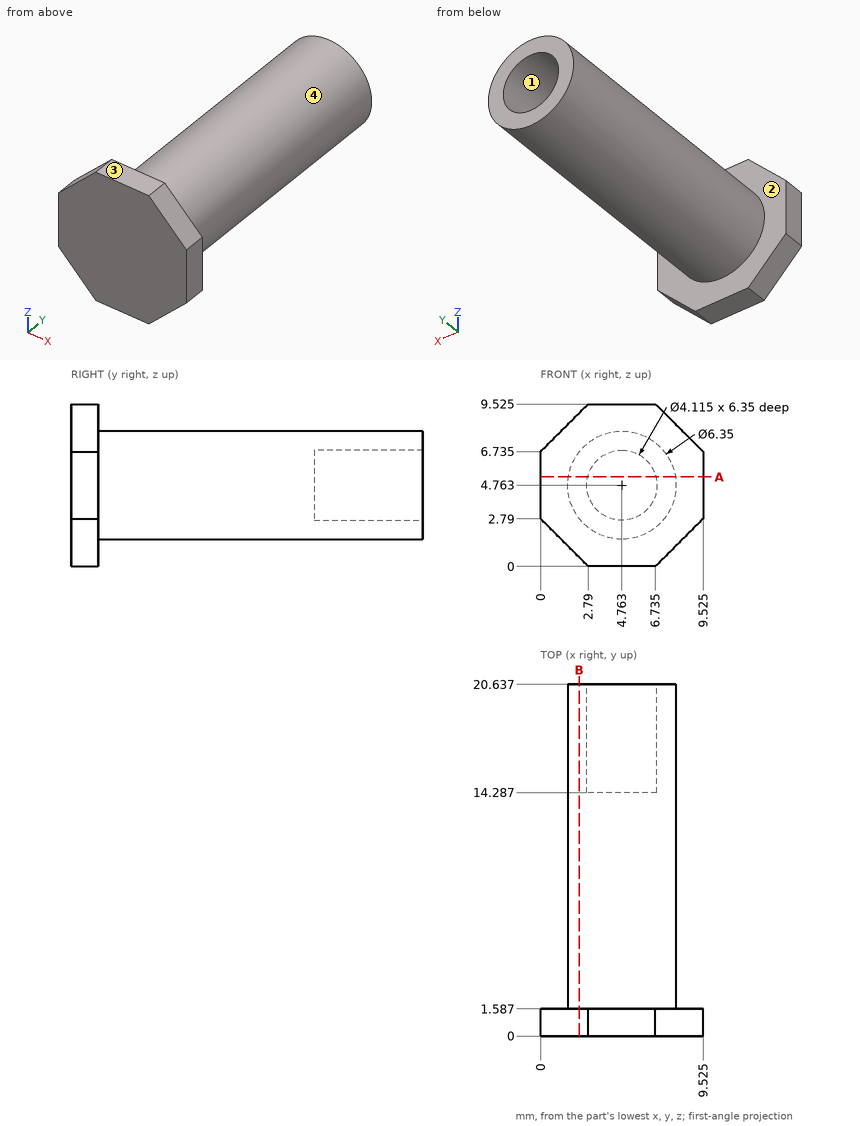
Geometry check sheet. Reference: drawing and pictorial views, mm from the part's lowest x, y, z. Give positions to 0.01 mm unless a question says otherwise; leave off trailing zeros. Order: outer loops, then holes, each group sorted by start corner. A loop starts at its lowest first (then second) coordinate and runs counter-clockwise, first axis right, second up. Notation, with made-up numbers: M -22.5,-20 L 22.5,-20 A29 ccw 22.5,8 Z; hole C 0.25,-35.75 d1. An arc over 180 degrees is marked long. Answer in a Markdown table with one row per item.
1) Gauge pin test, flat ends, axial feed: P1, Ø4, axis at y = 13, z = 6.5, coming from the -X side; P2, Ø3, axis at x = 3, y = 17.5, coming from the -Z side; P3, Ø4, axis at y = 8.5, z = 1.5, coming from the -X side. Record the tip position at first contact, or that the pin passes through.
Filled sheet:
| item | result |
|---|---|
| P1 | stops at x = 1.59 |
| P2 | stops at z = 1.6 |
| P3 | stops at x = 1.85 |
2) Thickness scan on L1, parallel to Y at x = 1, z = 3.25; L2, parallel to Y at x = 6.25, z = 5; L3, parallel to Z at x = 6, y = 15.25 (1 decimal). Record the ranges inside material, lowest first. Write a range as [from, to].
Filled sheet:
| item | result |
|---|---|
| L1 | y = [0, 1.59] |
| L2 | y = [0, 14.29] |
| L3 | z = [1.8, 3.1], [6.4, 7.7] |
3) Cross-section at A-A, the plane z = 5.25. Enter the section's corners in (x, y) (1 decimal).
Filled sheet:
| item | result |
|---|---|
| outline | M 0,0 L 9.5,0 L 9.5,1.6 L 7.9,1.6 L 7.9,20.6 L 6.8,20.6 L 6.8,14.3 L 2.8,14.3 L 2.8,20.6 L 1.6,20.6 L 1.6,1.6 L 0,1.6 Z |
4) Release check for a two-part mould opening along Z. For the marked faces 1, 2, 3 and 4 record: +Z half, -Z half, draft (parallel to the pull), parting line (faces both ways), or undercut.
Filled sheet:
| item | result |
|---|---|
| face 1 | undercut |
| face 2 | draft |
| face 3 | +Z half |
| face 4 | parting line |
5) Cross-section at B-B, the plane x = 2.25. Enter the section's corners in (y, z) (1 decimal).
Filled sheet:
| item | result |
|---|---|
| outline | M 0,0.5 L 1.6,0.5 L 1.6,2.8 L 20.6,2.8 L 20.6,6.7 L 1.6,6.7 L 1.6,9 L 0,9 Z |
